For this review, take the finished solid that the model builds, in its own axes (mm). Coordinates: 2 decimals unless noted, no trailing zeros. Order: outer loops, then holes, each group sorted by start corner. A loop starts at its lowest first (then second) coordinate and runs counter-clockwise, first axis right, second up. Notation, with made-up numbers: (-34, 19.25) -> (11, 19.25) arc R7 ccw to (11, 29.25) -> close; hole circle Ø4 at (27.25, -2). An arc over 180 degrees is marked (long way). Write item = value, one per line. Start each with the question number.
1) Wall thickness on probe 1 along X at (y, z) = (2.2, -57.35); probe 2 along X at (y, z) = (1.7, 91.25); probe 3 along X at (y, z) = (3.5, 71): over which ranges is each line inside the solid? List them lowest first. Write a range as [from, to].
2) Consider section D-D on y = 2.7. State how many separate pieces and enclosed holes the cut face has, and give its area (3 significant figures).
3) Consider section A-A on x = -7.85. Give the boundary of the cut face in (y, z).
4) Consider section B-B on z = -44. Give the boundary of the cut face in (x, y).
5) Consider section C-C on z = 111.25. Give the boundary of the cut face in (x, y), and give its area (3 significant figures).
6) Insertion check: pin 1 Ø1 at (y, z) = (1.5, 35) entering from +X; pin 2 Ø5.5 at (x, z) = (-7.85, 111.25) entering from -Y. Each pin has a flat end and moves straight along its axis. Give the tip position at first contact, or say it passes through.
from build123d import *

# Parameters (mm, degrees)
SKETCH1_W           = 75.7
SKETCH1_H           = 42.7
SKETCH1_R           = 1.75
BOSS_EXTRUDE1_DEPTH = 4
SKETCH3_W           = 75.7
SKETCH3_H           = 29.75
SKETCH3_R           = 1.75
BOSS_EXTRUDE2_DEPTH = 4
SKETCH3_3_R         = 1.75
CUT_EXTRUDE1_DEPTH  = 4
SKETCH4_W           = 75.7
SKETCH4_H           = 43.4
SKETCH4_R           = 1.75
BOSS_EXTRUDE3_DEPTH = 4
BOSS_EXTRUDE4_DEPTH = 4
SKETCH6_3_R         = 1.75
CUT_EXTRUDE2_DEPTH  = 111.432105839
SKETCH7_W           = 19.15
SKETCH7_H           = 10
SKETCH7_R           = 1.75
BOSS_EXTRUDE5_DEPTH = 4
SKETCH8_W           = 75.7
SKETCH8_H           = 21.5
BOSS_EXTRUDE6_DEPTH = 4
SKETCH9_R           = 1.75
CUT_EXTRUDE3_DEPTH  = 130.309705746
BOSS_EXTRUDE7_DEPTH = 4
CUT_EXTRUDE4_DEPTH  = 4
SKETCH12_W          = 10
SKETCH12_H          = 25
CUT_EXTRUDE5_DEPTH  = 10
SKETCH13_R          = 1.75
BOSS_EXTRUDE8_DEPTH = 4


with BuildPart() as part:
    # Sketch1 → Boss-Extrude1 (new body)
    with BuildSketch(Plane(origin=(0, 0, 0), x_dir=(1, 0, 0), z_dir=(0, 1, 0))):
        Rectangle(SKETCH1_W, SKETCH1_H)
        with Locations(Location((2.4, 17.25, 0), (0, 0, 270))):
            Circle(SKETCH1_R, mode=Mode.SUBTRACT)
        with Locations(Location((-33.8, -17.05, 0), (0, 0, 270))):
            Circle(SKETCH1_R, mode=Mode.SUBTRACT)
        with Locations(Location((29.5, -17.05, 0), (0, 0, 270))):
            Circle(SKETCH1_R, mode=Mode.SUBTRACT)
        with Locations(Location((33.9, 17.25, 0), (0, 0, 270))):
            Circle(SKETCH1_R, mode=Mode.SUBTRACT)
    extrude(amount=BOSS_EXTRUDE1_DEPTH)

    # Sketch3 → Boss-Extrude2 (add)
    # profile 1 of 2: a face of its own
    with BuildSketch(Plane(origin=(0, 4, 0), x_dir=(1, 0, 0), z_dir=(0, 1, 0))):
        with Locations((0, -36.225)):
            Rectangle(SKETCH3_W, SKETCH3_H)
        with Locations(Location((-2.1, -42.2, 0), (0, 0, 270))):
            Circle(SKETCH3_R, mode=Mode.SUBTRACT)
        with Locations(Location((-2.1, -27.2, 0), (0, 0, 270))):
            Circle(SKETCH3_R, mode=Mode.SUBTRACT)
    # profile 2 of 2: a face of its own
    with BuildSketch(Plane(origin=(0, 4, 0), x_dir=(1, 0, 0), z_dir=(0, 1, 0))):
        with BuildLine():
            Line((-2.1, -25.45), (-2.1, -21.35))
            Line((-2.1, -21.35), (-37.85, -21.35))
            Line((-37.85, -21.35), (-37.85, -51.1))
            Line((-37.85, -51.1), (-2.1, -51.1))
            Line((-2.1, -51.1), (-2.1, -43.95))
            ThreePointArc((-2.1, -43.95), (-3.85, -42.2), (-2.1, -40.45))
            Line((-2.1, -40.45), (-2.1, -28.95))
            ThreePointArc((-2.1, -28.95), (-3.85, -27.2), (-2.1, -25.45))
        make_face()
    extrude(amount=-BOSS_EXTRUDE2_DEPTH)

    # Sketch3<3> → Cut-Extrude1 (cut)
    with BuildSketch(Plane(origin=(0, 4, 0), x_dir=(1, 0, 0), z_dir=(0, 1, 0))):
        with Locations(Location((-2.1, 5.6, 0), (0, 0, 270))):
            Circle(SKETCH3_3_R)
        with Locations(Location((-2.1, -9.4, 0), (0, 0, 270))):
            Circle(SKETCH3_3_R)
    extrude(amount=-CUT_EXTRUDE1_DEPTH, mode=Mode.SUBTRACT)

    # Sketch4 → Boss-Extrude3 (add)
    # profile 1 of 2: a face of its own
    with BuildSketch(Plane(origin=(0, 0, 0), x_dir=(1, 0, 0), z_dir=(0, 1, 0))):
        with Locations((0, -72.8)):
            Rectangle(SKETCH4_W, SKETCH4_H)
        with Locations(Location((-32.85, -54.35, 0), (0, 0, 270))):
            Circle(SKETCH4_R, mode=Mode.SUBTRACT)
        with Locations(Location((-17.85, -54.35, 0), (0, 0, 270))):
            Circle(SKETCH4_R, mode=Mode.SUBTRACT)
        with Locations(Location((-17.85, -91.25, 0), (0, 0, 270))):
            Circle(SKETCH4_R, mode=Mode.SUBTRACT)
        with Locations(Location((-32.85, -91.25, 0), (0, 0, 270))):
            Circle(SKETCH4_R, mode=Mode.SUBTRACT)
        with Locations(Location((32.85, -91.25, 0), (0, 0, 90))):
            Circle(SKETCH4_R, mode=Mode.SUBTRACT)
        with Locations(Location((17.85, -91.25, 0), (0, 0, 90))):
            Circle(SKETCH4_R, mode=Mode.SUBTRACT)
        with Locations(Location((17.85, -54.35, 0), (0, 0, 90))):
            Circle(SKETCH4_R, mode=Mode.SUBTRACT)
        with Locations(Location((32.85, -54.35, 0), (0, 0, 90))):
            Circle(SKETCH4_R, mode=Mode.SUBTRACT)
    # profile 2 of 2: a face of its own
    with BuildSketch(Plane(origin=(0, 0, 0), x_dir=(1, 0, 0), z_dir=(0, 1, 0))):
        Polygon((-37.85, 21.35), (-44, 21.35), (-44, 29.35), (44, 29.35), (44, 21.35), (37.85, 21.35), align=None)
    extrude(amount=BOSS_EXTRUDE3_DEPTH)

    # Sketch6 → Boss-Extrude4 (add)
    with BuildSketch(Plane(origin=(0, 4, 0), x_dir=(1, 0, 0), z_dir=(0, 1, 0))):
        Polygon((-57, 31.35), (-57, 29.35), (-57, 21.35), (-44, 21.35), (-44, 26.251387819), (-44, 29.35), (44, 29.35), (44, 26.251387819), (44, 21.35), (57, 21.35), (57, 29.35), (57, 31.35), align=None)
    extrude(amount=-BOSS_EXTRUDE4_DEPTH)

    # Sketch6<3> → Cut-Extrude2 (cut, through all)
    with BuildSketch(Plane(origin=(0, 4, 0), x_dir=(1, 0, 0), z_dir=(0, 1, 0))):
        with Locations(Location((0, 27.35, 0), (0, 0, 270))):
            Circle(SKETCH6_3_R)
        with Locations(Location((20.5, 27.35, 0), (0, 0, 270))):
            Circle(SKETCH6_3_R)
        with Locations(Location((41, 27.35, 0), (0, 0, 270))):
            Circle(SKETCH6_3_R)
        with Locations(Location((-20.5, 27.35, 0), (0, 0, 270))):
            Circle(SKETCH6_3_R)
        with Locations(Location((-41, 27.35, 0), (0, 0, 270))):
            Circle(SKETCH6_3_R)
    extrude(amount=-CUT_EXTRUDE2_DEPTH, mode=Mode.SUBTRACT)

    # Sketch7 → Boss-Extrude5 (add)
    # profile 1 of 2: a face of its own
    with BuildSketch(Plane(origin=(0, 0, 0), x_dir=(1, 0, 0), z_dir=(0, 1, 0))):
        with Locations((-47.425, 16.35)):
            Rectangle(SKETCH7_W, SKETCH7_H)
        with Locations(Location((-52.5, 16.35, 0), (0, 0, 270))):
            Circle(SKETCH7_R, mode=Mode.SUBTRACT)
    # profile 2 of 2: a face of its own
    with BuildSketch(Plane(origin=(0, 0, 0), x_dir=(1, 0, 0), z_dir=(0, 1, 0))):
        with Locations((47.425, 16.35)):
            Rectangle(SKETCH7_W, SKETCH7_H)
        with Locations(Location((52.5, 16.35, 0), (0, 0, 270))):
            Circle(SKETCH7_R, mode=Mode.SUBTRACT)
    extrude(amount=BOSS_EXTRUDE5_DEPTH)

    # Sketch8 → Boss-Extrude6 (add)
    with BuildSketch(Plane(origin=(0, 0, 0), x_dir=(1, 0, 0), z_dir=(0, 1, 0))):
        with Locations((0, -105.25)):
            Rectangle(SKETCH8_W, SKETCH8_H)
    extrude(amount=BOSS_EXTRUDE6_DEPTH)

    # Sketch9 → Cut-Extrude3 (cut, through all)
    with BuildSketch(Plane(origin=(0, 4, 0), x_dir=(1, 0, 0), z_dir=(0, 1, 0))):
        with Locations(Location((-7.85, -111.25, 0), (0, 0, 270))):
            Circle(SKETCH9_R)
        with Locations(Location((-32.85, -111.25, 0), (0, 0, 270))):
            Circle(SKETCH9_R)
    cut_extrude3 = extrude(amount=-CUT_EXTRUDE3_DEPTH, mode=Mode.SUBTRACT)

    # Mirror1: Cut-Extrude3 across plane
    add(cut_extrude3.mirror(Plane(origin=(0, 0, 0), x_dir=(0, 0, 1), z_dir=(1, 0, 0))), mode=Mode.SUBTRACT)

    # Sketch10 → Boss-Extrude7 (add)
    with BuildSketch(Plane(origin=(0, 4, 0), x_dir=(1, 0, 0), z_dir=(0, 1, 0))):
        Polygon((-57, 11.35), (-37.85, -43.65), (-37.85, 11.35), align=None)
        Polygon((57, 11.35), (37.85, -43.65), (37.85, 11.35), align=None)
    extrude(amount=-BOSS_EXTRUDE7_DEPTH)

    # Sketch11 → Cut-Extrude4 (cut)
    with BuildSketch(Plane(origin=(0, 4, 0), x_dir=(1, 0, 0), z_dir=(0, 1, 0))):
        Polygon((-38.5, 11.35), (-13.5, 11.35), (-13.5, -48.65), align=None)
        Polygon((10, 11.35), (35, 11.35), (10, -48.65), align=None)
    extrude(amount=-CUT_EXTRUDE4_DEPTH, mode=Mode.SUBTRACT)

    # Sketch12 → Cut-Extrude5 (cut)
    with BuildSketch(Plane(origin=(0, 4, 0), x_dir=(1, 0, 0), z_dir=(0, 1, 0))):
        with Locations((0, -74.35)):
            Rectangle(SKETCH12_W, SKETCH12_H)
    extrude(amount=-CUT_EXTRUDE5_DEPTH, mode=Mode.SUBTRACT)

    # Sketch13 → Boss-Extrude8 (add)
    with BuildSketch(Plane(origin=(0, 0, 0), x_dir=(1, 0, 0), z_dir=(0, 1, 0))):
        Polygon((-57, 31.35), (-57, 50.810693545), (-45, 63.35), (45, 63.35), (57, 50.810693545), (57, 31.35), (50, 31.35), (50, 50.657737172), (47.423529439, 53.35), (-47.423529439, 53.35), (-50, 50.657737172), (-50, 31.35), align=None)
        with Locations(Location((-41, 57.35, 0), (0, 0, 270))):
            Circle(SKETCH13_R, mode=Mode.SUBTRACT)
        with Locations(Location((-20.5, 57.35, 0), (0, 0, 270))):
            Circle(SKETCH13_R, mode=Mode.SUBTRACT)
        with Locations(Location((0, 57.35, 0), (0, 0, 270))):
            Circle(SKETCH13_R, mode=Mode.SUBTRACT)
        with Locations(Location((20.5, 57.35, 0), (0, 0, 270))):
            Circle(SKETCH13_R, mode=Mode.SUBTRACT)
        with Locations(Location((41, 57.35, 0), (0, 0, 270))):
            Circle(SKETCH13_R, mode=Mode.SUBTRACT)
    extrude(amount=BOSS_EXTRUDE8_DEPTH)


solid = part.part
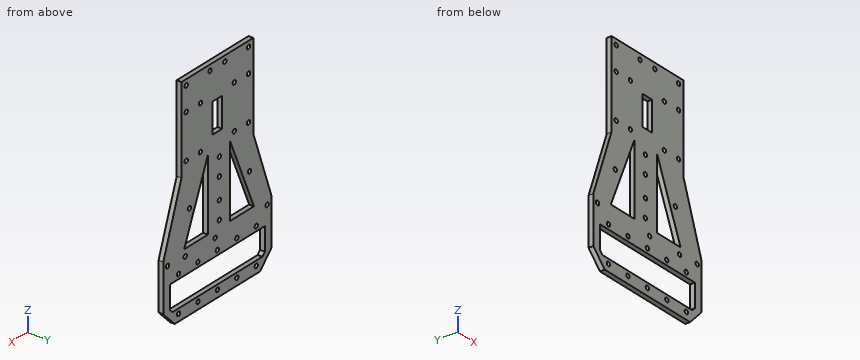
Answer sheet:
q1.probe_1 = [-50.74, -42.75], [-39.25, -22.25], [-18.75, -1.75], [1.75, 18.75], [22.25, 39.25], [42.75, 50.74]
q1.probe_2 = [-37.85, -34.6], [-31.1, -19.6], [-16.1, 16.1], [19.6, 31.1], [34.6, 37.85]
q1.probe_3 = [-37.85, -5], [5, 37.85]
q2.separate_pieces = 1
q2.enclosed_holes = 36
q2.area = 12,200 mm2
q3.outline = (0, -63.35) -> (4, -63.35) -> (4, -53.35) -> (0, -53.35) -> close; (0, -31.35) -> (4, -31.35) -> (4, 109.5) -> (0, 109.5) -> close; (0, 113) -> (4, 113) -> (4, 116) -> (0, 116) -> close
q4.outline = (-57, 0) -> (-50, 0) -> (-50, 4) -> (-57, 4) -> close; (50, 0) -> (57, 0) -> (57, 4) -> (50, 4) -> close
q5.outline = (-37.85, 0) -> (-34.6, 0) -> (-34.6, 4) -> (-37.85, 4) -> close; (-31.1, 0) -> (-9.6, 0) -> (-9.6, 4) -> (-31.1, 4) -> close; (-6.1, 0) -> (6.1, 0) -> (6.1, 4) -> (-6.1, 4) -> close; (9.6, 0) -> (31.1, 0) -> (31.1, 4) -> (9.6, 4) -> close; (34.6, 0) -> (37.85, 0) -> (37.85, 4) -> (34.6, 4) -> close
q5.area = 247 mm2
q6.pin_1 = 41.04
q6.pin_2 = 0
